Design review of the part shown in the three views and the two pictorial views. Dimensions are in mm from the part's minimum x, y and z. Give positions to 0.01 mm unless a question says otherwise; leave off trailing zeros. Order: outer loops, then holes, each group sorted by start corner. A loop starts at its lowest first (then second) coordinate and runs counter-clockwise, first axis right, second up. Notation, with made-up numbers: (35, -7.75) - (66, -7.75) arc R21 cw to (66, 0.25) - close; hole circle Ø9 at (24, 5.5). An arc over 180 degrees is marked (long way). Put each result on its own line as item: value.
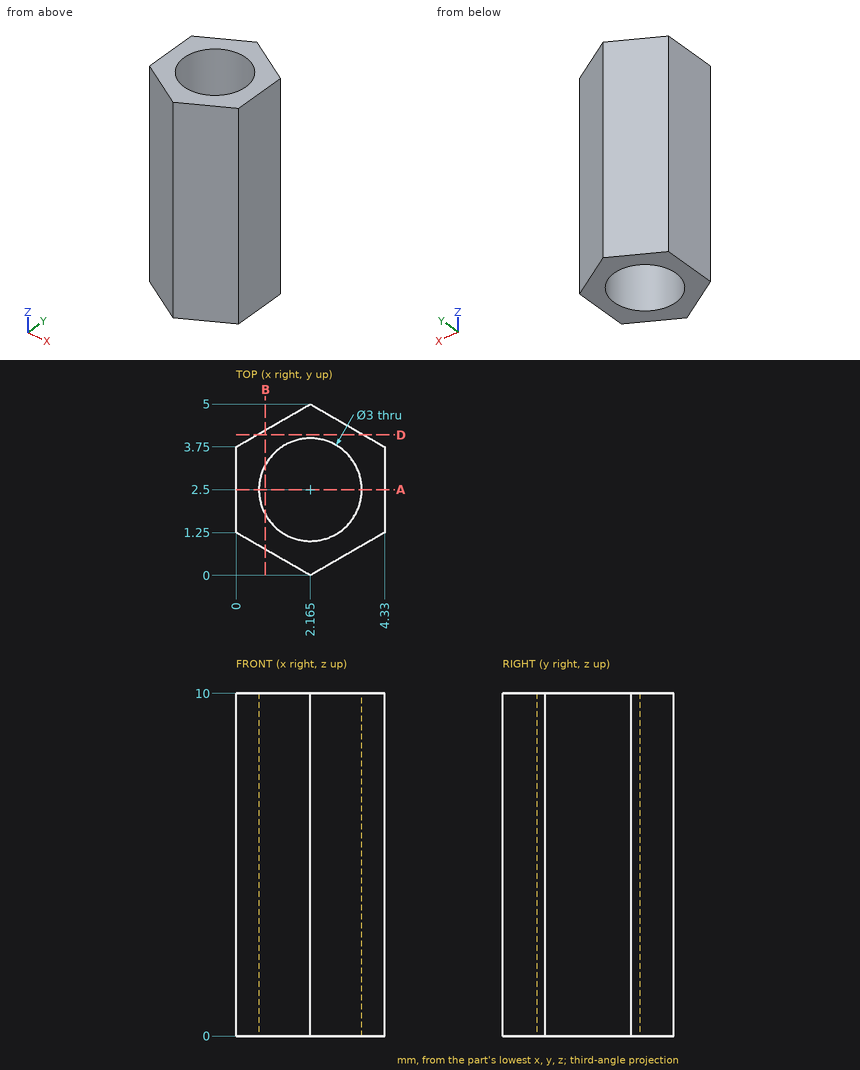
(1) Wall thickness on L1, parallel to Y at x = 2.95, z = 5; L2, parallel to Y at x = 1.65, z = 7; L3, parallel to X at y = 1.3, z = 1 (1 decimal): over which ranges is each line inside the solid? List them lowest first.
The answers:
L1: 0.45 to 1.22, 3.78 to 4.55
L2: 0.3 to 1.09, 3.91 to 4.7
L3: 0 to 1.3, 3.1 to 4.3
(2) Take a section at B-B, the plane x = 0.85. Write out the cut boundary in (y, z).
The answers:
outline: (0.76, 0) - (1.78, 0) - (1.78, 10) - (0.76, 10) - close; (3.22, 0) - (4.24, 0) - (4.24, 10) - (3.22, 10) - close
(3) Take a section at D-D, the plane y = 4.1. Write out the cut boundary in (x, z), then the cut area to 3 significant figures.
The answers:
outline: (0.61, 0) - (3.72, 0) - (3.72, 10) - (0.61, 10) - close
area: 31.2 mm^2
(4) Clearance check with a flat-ended pin moving along its axis: pin 1 Ø2 at (x, z) = (1, 2) entering from -Y (1 decimal). State where the tip first meets the part, or that it passes through.
The answers:
pin 1: y = 0.1
(5) Take a section at A-A, the plane y = 2.5. Write out the cut boundary in (x, z) (1 decimal).
The answers:
outline: (0, 0) - (0.7, 0) - (0.7, 10) - (0, 10) - close; (3.7, 0) - (4.3, 0) - (4.3, 10) - (3.7, 10) - close
